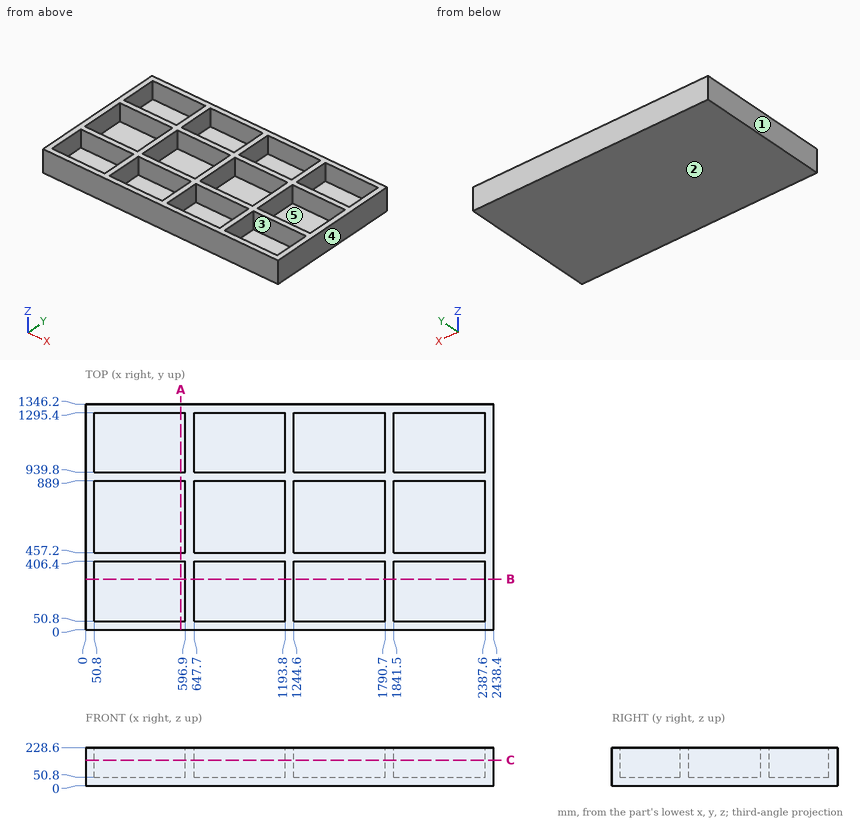
Could you check a few things on this drawing? It's one solid part, dimensions in mm from its lowest x, y, z. A direction names the side the tool comes from. Coordinates: 2 decimals unless noted, no trailing zeros. Write each loop counter-clockwise with the first axis right and the second up, starting at its lowest first coordinate (ties: lowest second). Pieces come first, ordered by that corner, then holes. Notation, with made-up numbers: (88.5, 25.25) - (93.5, 25.25) arc R11 ccw to (93.5, 30.25) - close; hole circle Ø11 at (59.25, 43). An arc over 180 degrees is marked (long way). Write item = value, one per line.
1) Please list where these lines run through material, in increasing order: line 1 (X direction, y = 1286, z = 72); line 2 (Y direction, x = 847, z = 124); line 3 (Z direction, x = 1763.5, y = 103.5). Write a range as [from, to].
Result set:
line_1 = [0, 50.8], [596.9, 647.7], [1193.8, 1244.6], [1790.7, 1841.5], [2387.6, 2438.4]
line_2 = [0, 50.8], [406.4, 457.2], [889, 939.8], [1295.4, 1346.2]
line_3 = [0, 50.8]
2) For the marked faces 4 and 5, which set-ups out of +Z, -Z, +X, -X, +Y, -Y let a thin tool reach every point of the face, with its end or its side?
Result set:
face_4 = +Z, -Z, +X, +Y, -Y
face_5 = +Z
3) Suppose I cut it at B-B on y = 301.5. Please give me the cut outline in (x, z), plus the area to 3 significant figures.
Result set:
outline = (0, 0) - (2438.4, 0) - (2438.4, 228.6) - (2387.6, 228.6) - (2387.6, 50.8) - (1841.5, 50.8) - (1841.5, 228.6) - (1790.7, 228.6) - (1790.7, 50.8) - (1244.6, 50.8) - (1244.6, 228.6) - (1193.8, 228.6) - (1193.8, 50.8) - (647.7, 50.8) - (647.7, 228.6) - (596.9, 228.6) - (596.9, 50.8) - (50.8, 50.8) - (50.8, 228.6) - (0, 228.6) - close
area = 169,000 mm2
4) Suppose I cut it at A-A on x = 569.5. Please give me the cut outline in (y, z).
Result set:
outline = (0, 0) - (1346.2, 0) - (1346.2, 228.6) - (1295.4, 228.6) - (1295.4, 50.8) - (939.8, 50.8) - (939.8, 228.6) - (889, 228.6) - (889, 50.8) - (457.2, 50.8) - (457.2, 228.6) - (406.4, 228.6) - (406.4, 50.8) - (50.8, 50.8) - (50.8, 228.6) - (0, 228.6) - close
5) Suppose I cut it at C-C on z = 153. State how many separate pieces and enclosed holes the cut face has, plus the area to 3 significant figures.
Result set:
separate_pieces = 1
enclosed_holes = 12
area = 786,000 mm2
6) We'd pull the mould along X, two halves only. Please class the marked faces 1, 2 and 3: +X half, -X half, draft (parallel to the pull), parting line (faces both ways), or undercut.
Result set:
face_1 = -X half
face_2 = draft
face_3 = undercut
